Autodesk Inventor part; units mm, degrees
ref_plane "YZ Plane" through (0, 0, 0) normal (1, 0, 0) x (0, 1, 0)
ref_plane "XZ Plane" through (0, 0, 0) normal (0, 1, 0) x (-1, 0, 0)
ref_plane "XY Plane" through (0, 0, 0) normal (0, 0, 1) x (1, 0, 0)
sketch "Sketch2" plane through (0, 0, 0) normal (0, 0, 1) x (1, 0, 0)
  circle A0 centre (0, 0) radius 4.5085
  circle A1 centre (0, 0) radius 15.875
  dimension "d3" = 9.017
  dimension "d4" = 31.75
extrude "Extrusion2" add sketch "Sketch2" along normal blind 8.382
chamfer "Chamfer1" distance 2.159 angle 45 1 edges at (-4.5085, 0, 8.382)
sketch "Sketch6" plane through (0, 0, 0) normal (0, 1, 0) x (-1, 0, 0)
  line L0 (15.875, 8.382) -> (-15.875, 8.382)
  line L1 (-15.875, 0) -> (15.875, 0)
  line L2 (15.875, 8.382) -> (12.7, 8.382)
  line L3 (15.875, 8.382) -> (-15.875, 8.382)
  line L4 (15.875, 8.382) -> (15.875, 6.9533)
  line L5 (15.875, 0) -> (15.875, 8.382)
  line L6 (15.875, 6.9533) -> (13.335, 6.9533)
  line L7 (13.335, 6.9533) -> (12.7, 8.382)
  line L8 (0, 0) -> (0, 8.967)
  dimension "d21" = 3.175
  dimension "d22" = 1.4287
  dimension "d23" = 2.54
revolve "Revolution1" cut sketch "Sketch6" angle 360 about axis through (0, 0, 0) along (0, 0, 1) contours L4 L6 L7 L0
sketch "Sketch7" plane through (0, 0, 0) normal (0, 0, -1) x (-1, 0, 0)
  line L0 (-3.3729, 8.3312) -> (-1.6864, 11.2522)
  line L1 (-1.6864, 11.2522) -> (1.6864, 11.2522)
  line L2 (1.6864, 11.2522) -> (3.3729, 8.3312)
  line L3 (3.3729, 8.3312) -> (1.6864, 5.4102)
  line L4 (1.6864, 5.4102) -> (-1.6864, 5.4102)
  line L5 (-1.6864, 5.4102) -> (-3.3729, 8.3312)
  point P0 (0, 0)
  point P1 (0, 8.3312)
  dimension "d27" = 8.3312
  dimension "d28" = 5.842
extrude "Extrusion4" cut sketch "Sketch7" against normal blind 4.064
chamfer "Chamfer3" distance 1.27 angle 45 6 edges at (2.5297, 9.7917, 4.064) (0, 11.2522, 4.064) (-2.5297, 9.7917, 4.064) (-2.5297, 6.8707, 4.064) (0, 5.4102, 4.064) (2.5297, 6.8707, 4.064)
pattern_circular "Circular Pattern1" count 3 over 360 about axis through (0, 0, 0) along (0, 0, 1) of "Extrusion4", "Chamfer3"
fillet "Fillet3" radius 3.175 1 edges at (13.335, 0, 6.9533)
properties part number "SpurGearThrustDistributer" material "ABS Plastic"
Design review of the part built by this model. Coordinates are the model's own, in mm. Coordinates: 2 decimals unless noted, no trailing zeros. Order: outer loops, then holes, each group sorted by start corner. A loop starts at its lowest first (then second) coordinate and runs counter-clockwise, first axis right, second up. Notation, with made-up numbers: (15.25, 42) -> (33.25, 42) arc R32 ccw to (33.25, 74) -> close; hole circle Ø2 at (67, -36). An arc over 180 degrees is marked (long way). One line per item, written item: value.
1) We need section C-C, the plane z = 3.5. Count the separate pieces of the cut face and the enclosed holes in it, then the cut area to 3 significant figures.
Output values:
separate pieces: 1
enclosed holes: 4
area: 677 mm2
2) To check wall thickness, follow probe 1 along Y at (x, z) = (0, 1.75) (1 decimal); probe 2 along X at (y, z) = (-6.5, 1.75); probe 3 along Y at (x, z) = (-2.5, 3). State the ranges of each line that lie inside material, in increasing order. Write a range as [from, to].
Output values:
probe 1: y = [-15.9, -4.5], [4.5, 5.4], [11.3, 15.9]
probe 2: x = [-14.48, -9.24], [-5.19, 5.19], [9.24, 14.48]
probe 3: y = [-15.68, -3.75], [3.75, 7.23], [9.43, 15.68]
3) We need section D-D, the plane z = 7.75. Give the boundary of the cut face in (x, y).
Output values:
outline: circle Ø26.5 at (0, 0); hole circle Ø12.07 at (0, 0)
4) Clearance check with flat-ended pins moving along their axes: P1, Ø3, axis at x = 6.5, z = 1, coming from the +Y side; P2, Ø1, axis at y = 9, z = 5.5, coming from the -X side; P3, Ø0.8, axis at x = -8, z = 1, coming from the -Y side. State where each tip first meets the part, or that it passes through.
Output values:
P1: stops at y = 15.07
P2: stops at x = -13.41
P3: stops at y = -13.94
5) Draft analysis for pull direction X (two halves, no side actions). For faces 1 (the face through (1.98, 9.45, 3.44)), 2 (the face through (5, -5, 8.382)), state which applies: +X half, -X half, draft (parallel to the pull), parting line (faces both ways), or undercut.
Output values:
face 1: undercut
face 2: draft
